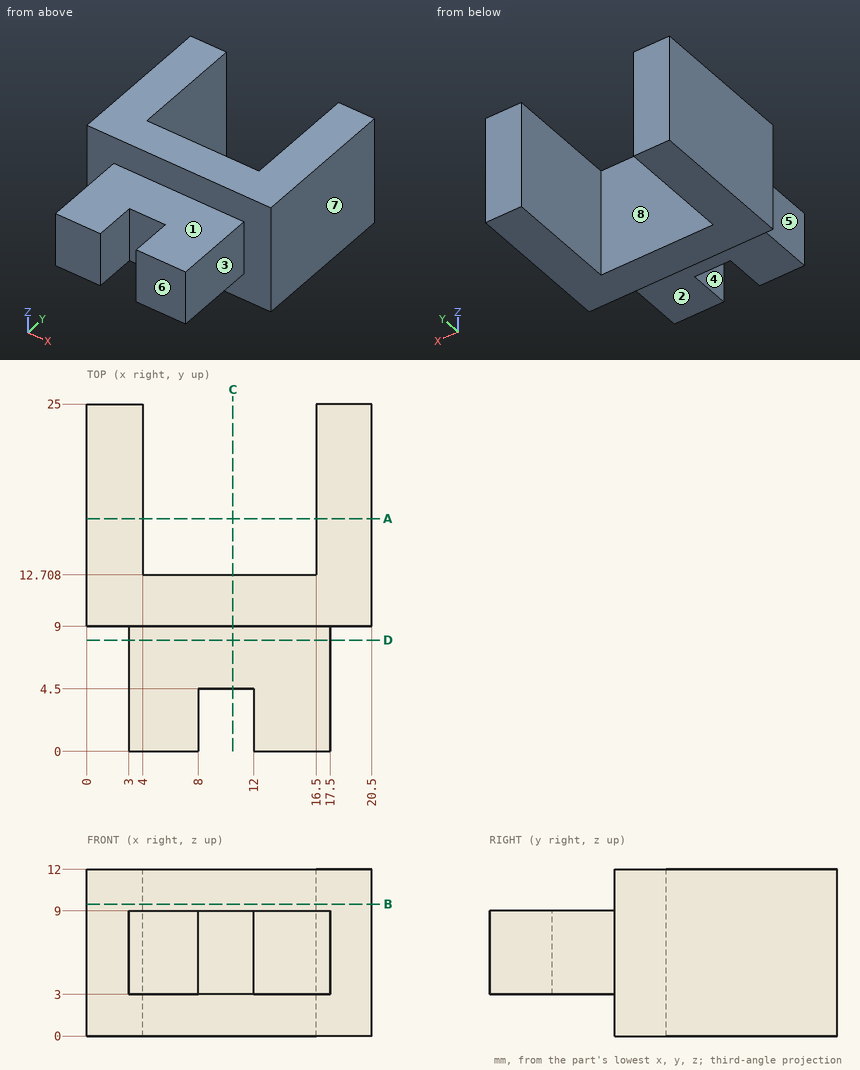
Study the drawing (mm; zero at the part's minimum x, y, z) and answer. A direction names the side the tool comes from. Give positions to 0.01 mm unless a question says otherwise; leave off trailing zeros. Loops run counter-clockwise (first coordinate to the right, second up) from the corner with the lowest first, then second, coordinate; pieces in that order, holes last. Notation, with made-up numbers: (-7.75, 74) -> (33.25, 74) arc R30 ccw to (33.25, 112) -> close; hole circle Ø5 at (49.5, 20.5). An arc over 180 degrees is marked (long way). Use a Markdown table: item, result. Add a question column.
1) Each of these flat-tipped pins is pushed along its axis until it touches: P1, Ø5, axis at x = 14.5, z = 6, coming from the -Y side; P2, Ø1.8, axis at y = 5.5, z = 6, coming from the -X side; P3, Ø1.3, axis at y = 2.5, z = 6.5, coming from the +X side; P4, Ø3, axis at x = 8.5, y = 6.5, coming from the +Z side. Where does it stop, or does it pass through?
2) Consider line 1 along X through (y, z) = (20.5, 8); line 2 along Z through (x, y) = (7.5, 2); line 3 along X through (y, z) = (7, 4.25). Determine where each line is inside the solid, lowest interval first.
3) The part is cut by section D-D, the plane y = 8. Determine the outline of the cut face in (x, z).
4) The part is cut by section A-A, the plane y = 16.75. Determine the outline of the cut face in (x, z), plus the area to 3 significant figures.
5) The part is cut by section B-B, the plane z = 9.5. Determine the outline of the cut face in (x, y), plus the area to 3 significant figures.
6) For a pull along X with two mould halves and no side action, classify the marked faces 6, 7 and 8 as +X half, -X half, draft (parallel to the pull), parting line (faces both ways), or undercut.
7) Which of the six approach directions +Z, -Z, +X, -X, +Y, -Y give full straight-line access (tool end or side, diameter ignored) to the marked faces 1, 2, 3, 4 and 5?
8) The part is cut by section C-C, the plane x = 10.5. Determine the outline of the cut face in (y, z), plus the area to 3 significant figures.
Reported:
| question | item | result |
|---|---|---|
| 1 | P1 | stops at y = 0 |
| 1 | P2 | stops at x = 3 |
| 1 | P3 | stops at x = 17.5 |
| 1 | P4 | stops at z = 9 |
| 2 | line 1 | x = 0 to 4, 16.5 to 20.5 |
| 2 | line 2 | z = 3 to 9 |
| 2 | line 3 | x = 3 to 17.5 |
| 3 | outline | (3, 3) -> (17.5, 3) -> (17.5, 9) -> (3, 9) -> close |
| 4 | outline | (0, 0) -> (4, 0) -> (4, 12) -> (0, 12) -> close; (16.5, 0) -> (20.5, 0) -> (20.5, 12) -> (16.5, 12) -> close |
| 4 | area | 96.0 mm^2 |
| 5 | outline | (0, 9) -> (20.5, 9) -> (20.5, 25) -> (16.5, 25) -> (16.5, 12.71) -> (4, 12.71) -> (4, 25) -> (0, 25) -> close |
| 5 | area | 174 mm^2 |
| 6 | face 6 | draft |
| 6 | face 7 | +X half |
| 6 | face 8 | undercut |
| 7 | face 1 | +Z, +X, -X, -Y |
| 7 | face 2 | -Z, +X, -X, -Y |
| 7 | face 3 | +Z, -Z, +X, -Y |
| 7 | face 4 | +Z, -Z, -Y |
| 7 | face 5 | +Z, -Z, -X, -Y |
| 8 | outline | (4.5, 3) -> (9, 3) -> (9, 0) -> (12.71, 0) -> (12.71, 12) -> (9, 12) -> (9, 9) -> (4.5, 9) -> close |
| 8 | area | 71.5 mm^2 |
